```python
from build123d import *

# Parameters (mm, degrees)
SKETCH2_W          = 2.5
SKETCH2_H          = 1.2
SKETCH2_W_2        = 1.2
SKETCH2_H_2        = 2.5
CUT_EXTRUDE1_DEPTH = 4


with BuildPart() as part:
    # Sketch1 → Revolve1 (revolve)
    with BuildSketch(Plane(origin=(0, 0, 0), x_dir=(1, 0, 0), z_dir=(0, 1, 0))):
        with BuildLine():
            ThreePointArc((10, 48.210245834), (5.423494003, 45.101396028), (0, 44.008204805))
            Line((0, 44.008204805), (0, 43.710245834))
            Line((0, 43.710245834), (14, 43.710245834))
            Line((14, 43.710245834), (14, 48.710245834))
            Line((14, 48.710245834), (12, 48.710245834))
            Line((12, 48.710245834), (12, 48.210245834))
            Line((12, 48.210245834), (10, 48.210245834))
        make_face()
    revolve(axis=Axis((0, 0, -48.710245834), (0, 0, 1)))

    # Sketch2 → Cut-Extrude1 (cut)
    with BuildSketch(Plane(origin=(0, 0, -48.710245834), x_dir=(-1, 0, 0), z_dir=(0, 0, -1))):
        with Locations((0, 13)):
            Rectangle(SKETCH2_W, SKETCH2_H)
        with Locations((-13, 0)):
            Rectangle(SKETCH2_W_2, SKETCH2_H_2)
        with Locations((13, 0)):
            Rectangle(SKETCH2_W_2, SKETCH2_H_2)
        with Locations((0, -13)):
            Rectangle(SKETCH2_W, SKETCH2_H)
    extrude(amount=-CUT_EXTRUDE1_DEPTH, mode=Mode.SUBTRACT)


solid = part.part
```
Model file for the job. Use its own axes, mm. Round coordinates to 2 decimals unless told otherwise and drop trailing zeros. Write each loop counter-clockwise with the first axis right and the second up, starting at its lowest first coordinate (ties: lowest second). Pieces come first, ordered by that corner, then holes. Notation, with made-up numbers: (8, -14) - (20, -14) arc R9 cw to (20, -1) - close; hole circle Ø3 at (-38, 10). An arc over 180 degrees is marked (long way). Use CSV: the item, a comma, the result in double quotes. Start each with the question number.
Item 1: Band-saw the part on A-A (y = 0). Write the cut outline in (x, z).
Item 2: Drill centre lines: L1, parallel to Y at x = 0, z = -48.6; L2, parallel to Y at x = 0.75, z = -45.25; L3, parallel to X at y = 2.5, z = -45.4. Where is each one in solid material? Low to high. Write a range as [from, to].
Item 3: Pin check, flat tips, straight feed: P1, Ø0.6, axis at x = -13, z = -46, coming from the +Y side; P2, Ø1, axis at x = -13, y = 0.5, coming from the -Z side; P3, Ø1.3, axis at x = 12.5, z = -46, coming from the -Y side. Stop position of each tip, or through.
Item 4: Band-saw the part on C-C (z = -46.2). Write the cut outline in (x, y).
Item 5: Two-plate mould, pull along X, no slides. Class faces 1 (the face through (0, 0, -43.71)), 2 (the face through (-1.25, -13, -47)): released by +X, released by -X, zero draft, split by the parting line, or undercut.
Item 6: Band-saw the part on D-D (x = -3). Write the cut outline in (y, z).
Checked values:
1,outline,"(-14, -48.71) - (-13.6, -48.71) - (-13.6, -44.71) - (-12.4, -44.71) - (-12.4, -48.71) - (-12, -48.71) - (-12, -48.21) - (-10, -48.21) arc R14 cw to (10, -48.21) - (12, -48.21) - (12, -48.71) - (12.4, -48.71) - (12.4, -44.71) - (13.6, -44.71) - (13.6, -48.71) - (14, -48.71) - (14, -43.71) - (-14, -43.71) - close"
2,L1,"y = [-14, -13.6], [-12.4, -12], [12, 12.4], [13.6, 14]"
2,L2,"y = [-13.98, -13.6], [-12.4, -5.72], [5.72, 12.4], [13.6, 13.98]"
2,L3,"x = [-13.77, -5.55], [5.55, 13.77]"
3,P1,"stops at y = 5.89"
3,P2,"stops at z = -44.71"
3,P3,"stops at y = -7.46"
4,outline,"circle Ø28 at (0, 0); hole (-13.6, -1.25) - (-12.4, -1.25) - (-12.4, 1.25) - (-13.6, 1.25) - close; hole circle Ø15.04 at (0, 0); hole (-1.25, -13.6) - (1.25, -13.6) - (1.25, -12.4) - (-1.25, -12.4) - close; hole (-1.25, 12.4) - (1.25, 12.4) - (1.25, 13.6) - (-1.25, 13.6) - close; hole (12.4, -1.25) - (13.6, -1.25) - (13.6, 1.25) - (12.4, 1.25) - close"
5,face 1,"zero draft"
5,face 2,"undercut"
6,outline,"(-13.67, -48.71) - (-11.62, -48.71) - (-11.62, -48.21) - (-9.54, -48.21) arc R13.67 cw to (9.54, -48.21) - (11.62, -48.21) - (11.62, -48.71) - (13.67, -48.71) - (13.67, -43.71) - (-13.67, -43.71) - close"
